Autodesk Inventor part; units mm, degrees
ref_plane "YZ Plane" through (0, 0, 0) normal (1, 0, 0) x (0, 1, 0)
ref_plane "XZ Plane" through (0, 0, 0) normal (0, 1, 0) x (-1, 0, 0)
ref_plane "XY Plane" through (0, 0, 0) normal (0, 0, 1) x (1, 0, 0)
ref_plane "Work Plane2" through (0, 0, 0) normal (0, 0, 1) x (1, 0, 0)
sketch "Sketch2" plane through (0, 0, 0) normal (0, 0, 1) x (1, 0, 0)
  line L0 (-70.75, 49.5) -> (-69.25, 49.5) construction
  line L1 (-70.75, 39.5) -> (-70.75, 49.5) construction
  line L2 (-69.25, 39.5) -> (-70.75, 39.5) construction
  line L3 (-69.25, 49.5) -> (-69.25, 39.5) construction
  line L4 (-76.75, 49.5) -> (-75.25, 49.5) construction
  line L5 (-76.75, 39.5) -> (-76.75, 49.5) construction
  line L6 (-75.25, 39.5) -> (-76.75, 39.5) construction
  line L7 (-75.25, 39.5) -> (-75.25, 49.5) construction
  line L8 (-75.25, 44.5) -> (-70.75, 44.5) construction
  line L9 (-75.375, 39.5) -> (-75.375, 49.5)
  line L10 (-75.375, 49.5) -> (-70.625, 49.5) construction
  line L11 (-70.625, 49.5) -> (-70.625, 39.5)
  line L12 (-70.625, 39.5) -> (-75.375, 39.5)
  line L13 (-75.375, 39.5) -> (-70.625, 49.5) construction
  line L14 (-75.375, 49.5) -> (-70.625, 39.5) construction
  line L15 (-68, 37) -> (-78, 37)
  line L16 (-78, 37) -> (-78, 52)
  line L17 (-78, 52) -> (-75.375, 52)
  line L18 (-68, 52) -> (-68, 37)
  line L19 (-68, 37) -> (-78, 52) construction
  line L20 (-78, 37) -> (-68, 52) construction
  line L21 (-75.375, 49.5) -> (-75.375, 51)
  line L22 (-70.625, 49.5) -> (-70.625, 51)
  line L23 (-75.375, 52) -> (-70.625, 52) construction
  line L24 (-70.625, 52) -> (-68, 52)
  arc A0 (-75.375, 51) -> (-75.375, 52) centre (-75.375, 51.5) ccw
  arc A1 (-70.625, 52) -> (-70.625, 51) centre (-70.625, 51.5) ccw
  line L25 (-75.375, 51) -> (-75.375, 52) construction
  arc A2 (-75.375, 52) -> (-75.375, 51) centre (-75.375, 51.5) ccw construction
  arc A3 (-70.625, 51) -> (-70.625, 52) centre (-70.625, 51.5) ccw construction
  line L26 (-70.625, 51) -> (-70.625, 52) construction
  point P0 (0, 0)
  point P1 (-73, 44.5)
  dimension "d0" = 4.75
  dimension "d1" = 10
  dimension "d2" = 15
  dimension "d3" = 1
  dimension "d4" = 1
extrude "Extrusion1" add sketch "Sketch2" along normal blind 1.9
properties part number "IRHolder_new2"
Input: part model. Units: mm. Frame: model coordinates. A direction names the side the tool comes from. Coordinates: 2 decimals unless noted, no trailing zeros. Loops run counter-clockwise (first coordinate to the right, second up) from the corner with the lowest first, then second, coordinate; pieces in that order, holes last. Notation, with made-up numbers: (88.25, 51) -> (103.25, 51) arc R24 ccw to (103.25, 88) -> close; hole circle Ø7 at (17, 73.5). An arc over 180 degrees is marked (long way). Use a Markdown table: item, result.
1) Cut plane B-B (z = 0.3). Return the cut outline in (x, y) (3 decimals), then the cut area to 3 significant figures.
Results found:
| item | result |
|---|---|
| outline | (-78, 37) -> (-68, 37) -> (-68, 52) -> (-70.625, 52) arc R0.5 ccw to (-70.625, 51) -> (-70.625, 39.5) -> (-75.375, 39.5) -> (-75.375, 51) arc R0.5 ccw to (-75.375, 52) -> (-78, 52) -> close |
| area | 91.4 mm2 |
2) Access query for faces 4 (the flat face through (-70.625, 45, 1)), 5 (the flat face through (-70, 45, 0)). Directions: +Z, -Z, +X, -X, +Y, -Y. A direction counts if a zero-diameter tool reaches every point of the face in a straight line with its end or side. Return the directions, or none.
Results found:
| item | result |
|---|---|
| face 4 | +Z, -Z |
| face 5 | -Z, +X, -X, +Y, -Y |
3) Pull-direction query (X, two-part tool) for faces 1 (the flat face through (-73, 37, 1)), 2 (the flat face through (-68, 45, 1)), 3 (the flat face through (-73, 39.5, 1)); classes: released by +X, released by -X, zero draft, split by the parting line, or undercut.
Results found:
| item | result |
|---|---|
| face 1 | zero draft |
| face 2 | released by +X |
| face 3 | undercut |
4) Cut plane A-A (y = 41.5). Return the cut outline in (x, z) (3 decimals).
Results found:
| item | result |
|---|---|
| outline | (-78, 0) -> (-75.375, 0) -> (-75.375, 1.9) -> (-78, 1.9) -> close; (-70.625, 0) -> (-68, 0) -> (-68, 1.9) -> (-70.625, 1.9) -> close |
5) Material intervals for line 1 along X through (y, z) = (50, 0.9) (3 decimals); line 2 along Y through (x, z) = (-73, 1.3); line 3 along Y through (x, z) = (-75, 1.8), sorted ascending. Write a range as from..to.
Results found:
| item | result |
|---|---|
| line 1 | x = -78..-75.375, -70.625..-68 |
| line 2 | y = 37..39.5 |
| line 3 | y = 37..39.5, 51.17..51.83 |
6) Contact query for a flat-ended pin moving along its axis: pin 1 (0.6 mm diameter, centred on x = -74, z = 1, fed in from +Y). Output: stop coordinate, or through.
Results found:
| item | result |
|---|---|
| pin 1 | stops at y = 39.5 |
7) Cut plane C-C (y = 51.5). Return the cut outline in (x, z) (3 decimals).
Results found:
| item | result |
|---|---|
| outline | (-78, 0) -> (-74.875, 0) -> (-74.875, 1.9) -> (-78, 1.9) -> close; (-71.125, 0) -> (-68, 0) -> (-68, 1.9) -> (-71.125, 1.9) -> close |
